```python
from build123d import *

# Parameters (mm, degrees)
SKETCH1_R           = 12.5
BOSS_EXTRUDE1_DEPTH = 75
CUT_EXTRUDE1_DEPTH  = 65
CHAMFER1_SIZE       = 1.5
FILLET1_R           = 3
FILLET2_R           = 1


with BuildPart() as part:
    # Sketch1 → Boss-Extrude1 (new body)
    with BuildSketch(Plane.XY):
        Circle(SKETCH1_R)
    extrude(amount=BOSS_EXTRUDE1_DEPTH)

    # Sketch2 → Cut-Extrude1 (cut)
    with BuildSketch(Plane(origin=(0, 0, 0), x_dir=(-1, 0, 0), z_dir=(0, 0, -1))):
        with BuildLine():
            Line((-4.045894985, 8.5), (0, 8.5))
            Line((0, 8.5), (0, 12.5))
            ThreePointArc((0, 12.5), (-2.050733749, 12.330632226), (-4.045894985, 11.827118574))
            Line((-4.045894985, 11.827118574), (-4.045894985, 8.5))
        make_face()
        with BuildLine():
            Line((0, 12.5), (0, 8.5))
            Line((0, 8.5), (3.954105015, 8.5))
            Line((3.954105015, 8.5), (3.954105015, 11.858121838))
            ThreePointArc((3.954105015, 11.858121838), (2.002932478, 12.338487002), (0, 12.5))
        make_face()
    extrude(amount=-CUT_EXTRUDE1_DEPTH, mode=Mode.SUBTRACT)

    # Chamfer1
    chamfer1_edges = [part.edges().sort_by_distance(p)[0] for p in [
        (-7.308340691, -10.140914966, 0),
    ]]
    chamfer(chamfer1_edges, length=CHAMFER1_SIZE)

    # Fillet1
    fillet1_edges = [part.edges().sort_by_distance(p)[0] for p in [
        (0.045894985, 8.5, 65),
    ]]
    fillet(fillet1_edges, radius=FILLET1_R)

    # Fillet2
    fillet2_edges = [part.edges().sort_by_distance(p)[0] for p in [
        (-12.5, 0, 75),
    ]]
    fillet(fillet2_edges, radius=FILLET2_R)


solid = part.part
```
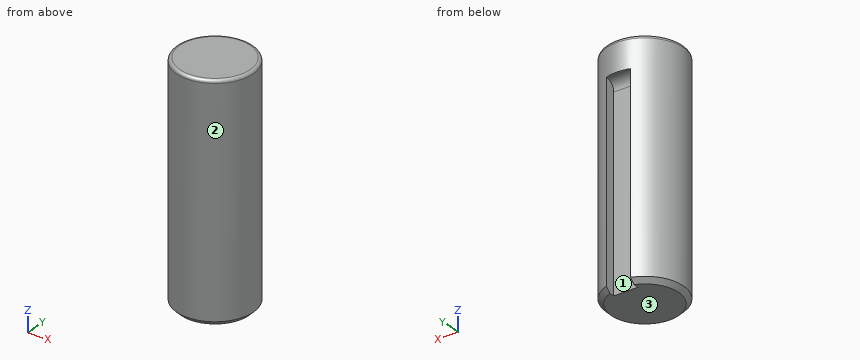
For this review, take the finished solid that the model builds, in its own axes (mm). Face numbers are marked on the shaded views. Coordinates: 2 decimals unless noted, no trailing zeros. Write each loop counter-clockwise with the first axis right and the second up, starting at its lowest first coordinate (ties: lowest second). Pieces come first, ordered by that corner, then holes. Notation, with made-up numbers: (-37, 44.25) - (14, 44.25) arc R21 cw to (14, 70.25) - close; hole circle Ø2 at (89, 78). An arc over 180 degrees is marked (long way). Answer in a Markdown table with one row per item. Add a question column.
Q1. We need section B-B, the plane z = 9.5. State the section outline as (x, y) points.
Q2. For probe 1 along X at (y, z) = (10.75, 44); probe 2 along X at (y, z) = (-0.25, 48); probe 3 along Y at (x, z) = (-0.5, 22), list the stretches that pass through material, from the lowest coordinate up.
Q3. We need section A-A, the plane x = 0. State the section outline as (y, z) points.
Q4. For P1, Ø0.5, axis at x = -2, y = 12, coming from the -Z side; P2, Ø9, axis at x = -1, z = 37.5, coming from the +Y side; P3, Ø1.5, axis at x = -3.5, z = 14.5, coming from the -Y side; P4, Ø6, axis at x = -2.5, y = 4, coming from the -Z side, all flat-tipped, find the tip position at first contact; note any pin that passes through.
Q5. Draft analysis for pull direction X (two halves, no side actions). For the marked faces 1, 2 and 3, state which applies: +X half, -X half, draft (parallel to the pull), parting line (faces both ways), or undercut.
Answer list:
| question | item | result |
|---|---|---|
| 1 | outline | (-3.95, 8.5) - (-3.95, 11.86) arc R12.5 ccw (long way) to (4.05, 11.83) - (4.05, 8.5) - close |
| 2 | probe 1 | x = -6.38 to -3.95, 4.05 to 6.38 |
| 2 | probe 2 | x = -12.5 to 12.5 |
| 2 | probe 3 | y = -12.49 to 8.5 |
| 3 | outline | (-12.5, 1.5) - (-11, 0) - (8.5, 0) - (8.5, 62) arc R3 cw to (11.5, 65) - (12.5, 65) - (12.5, 74) arc R1 ccw to (11.5, 75) - (-11.5, 75) arc R1 ccw to (-12.5, 74) - close |
| 4 | P1 | stops at z = 65 |
| 4 | P2 | stops at y = 11.86 |
| 4 | P3 | stops at y = -12.19 |
| 4 | P4 | stops at z = 0 |
| 5 | face 1 | undercut |
| 5 | face 2 | parting line |
| 5 | face 3 | draft |
